from build123d import *

# Parameters (mm, degrees)
F0_W     = 205.775664
F0_H     = 100
F0_R     = 25
F1_DEPTH = 50
F2_W     = 20
F2_H     = 100
F3_DEPTH = 10
F5_DEPTH = 100.001
F6_R     = 7.5
F7_DEPTH = 25


with BuildPart() as f1:
    # F0 (on Top) → F1 (new body)
    with BuildSketch(Plane.XY):
        Rectangle(F0_W, F0_H)
        Circle(F0_R, mode=Mode.SUBTRACT)
    extrude(amount=F1_DEPTH)

    # F2 (on face) → F3 (cut)
    with BuildSketch(Plane(origin=(0, 0, 0), x_dir=(1, 0, 0), z_dir=(0, 0, -1))):
        with Locations((-67.887832, 0)):
            Rectangle(F2_W, F2_H)
        with BuildLine():
            Line((11, 50), (-11, 50))
            Line((-11, 50), (-11, 22.449944))
            ThreePointArc((-11, 22.449944), (0, 25), (11, 22.449944))
            Line((11, 22.449944), (11, 50))
        make_face()
        with BuildLine():
            Line((-11, -22.449944), (-11, -50))
            Line((-11, -50), (11, -50))
            Line((11, -50), (11, -22.449944))
            ThreePointArc((11, -22.449944), (0, -25), (-11, -22.449944))
        make_face()
    extrude(amount=-F3_DEPTH, mode=Mode.SUBTRACT)

    # F4 (on face) → F5 (cut, through all)
    with BuildSketch(Plane(origin=(0, 50, 0), x_dir=(-1, 0, 0), z_dir=(0, 1, 0))):
        Polygon((-62.5, 0), (-37.5, 0), (-31.726497, 10), (-68.273503, 10), align=None)
    extrude(amount=-F5_DEPTH, mode=Mode.SUBTRACT)

    # F6 (on face) → F7 (join)
    with BuildSketch(Plane.YZ.offset(102.887832)):
        with Locations((0, 25)):
            Circle(F6_R)
    extrude(amount=F7_DEPTH)


solid = f1.part
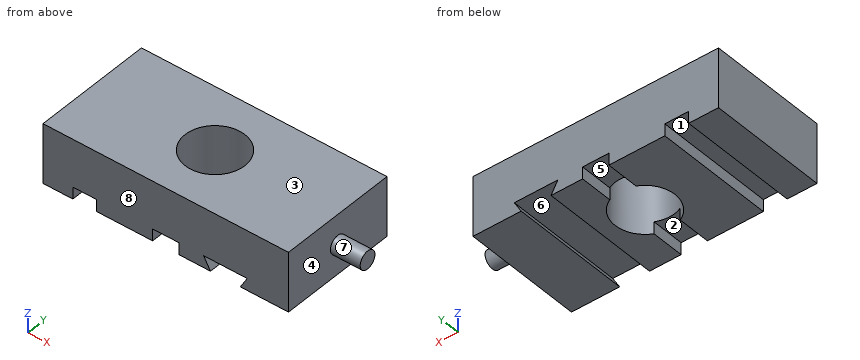
The listing builds one solid part. Answer for the finished solid, in the listing's coordinates (mm). Face numbers are marked on the shaded views. A direction names the side the tool comes from. Round coordinates to 2 decimals unless told otherwise and drop trailing zeros. Order: outer loops, then holes, each group sorted by start corner. A loop starts at its lowest first (then second) coordinate and runs counter-clockwise, first axis right, second up. Notation, with made-up numbers: (-14.75, 16.5) -> (0.25, 16.5) arc R12 cw to (0.25, 36.5) -> close; hole circle Ø1 at (86, 32.25). An arc over 180 degrees is marked (long way). Put each result on its own line as item: value.
Q1. Section D-D, the plane y = 42.5 is taken. Write down the section's boundary in (x, z).
Results list:
outline: (-102.89, 0) -> (-77.89, 0) -> (-77.89, 10) -> (-57.89, 10) -> (-57.89, 0) -> (-11, 0) -> (-11, 10) -> (11, 10) -> (11, 0) -> (37.5, 0) -> (31.73, 10) -> (68.27, 10) -> (62.5, 0) -> (102.89, 0) -> (102.89, 50) -> (-102.89, 50) -> close
Q2. Each of these flat-tipped pins is pushed along its axis until it touches: P1, Ø15, axis at y = 20.5, z = 17.5, coming from the +X side; P2, Ø1.5, axis at x = 40.5, y = -38, coming from the -Z side. Where does it stop, or does it pass through?
Results list:
P1: x = 102.89
P2: z = 10
Q3. Section A-A, the plane y = 0 is taken. Write down the section's boundary in (x, z).
Results list:
outline: (-102.89, 0) -> (-77.89, 0) -> (-77.89, 10) -> (-57.89, 10) -> (-57.89, 0) -> (-25, 0) -> (-25, 50) -> (-102.89, 50) -> close; (25, 0) -> (37.5, 0) -> (31.73, 10) -> (68.27, 10) -> (62.5, 0) -> (102.89, 0) -> (102.89, 17.5) -> (127.89, 17.5) -> (127.89, 32.5) -> (102.89, 32.5) -> (102.89, 50) -> (25, 50) -> close
Q4. Section B-B, the plane x = 0 is taken. Write down the section's boundary in (y, z), and give its area (3 significant figures).
Results list:
outline: (-50, 10) -> (-25, 10) -> (-25, 50) -> (-50, 50) -> close; (25, 10) -> (50, 10) -> (50, 50) -> (25, 50) -> close
area: 2,000 mm^2
Q5. Section C-C, the plane z = 25 is taken. Write down the section's boundary in (x, y).
Results list:
outline: (-102.89, -50) -> (102.89, -50) -> (102.89, -7.5) -> (127.89, -7.5) -> (127.89, 7.5) -> (102.89, 7.5) -> (102.89, 50) -> (-102.89, 50) -> close; hole circle Ø50 at (0, 0)
Q6. Which of the six approach directions +Z, -Z, +X, -X, +Y, -Y give full straight-line access (tool end or side, diameter ignored) to the marked faces 5, 6, 7 and 8?
Results list:
face 5: -Z, +Y, -Y
face 6: +Y, -Y
face 7: +X
face 8: +Z, -Z, +X, -X, -Y
Q7. Determine the mould class of the marked faces 1, 2, 3 and 4 for opening direction X: pulls with the +X half, pulls with the -X half, needs draft (parallel to the pull), parting line crosses it, or undercut.
Results list:
face 1: undercut
face 2: undercut
face 3: needs draft
face 4: pulls with the +X half
Q8. Consider line 1 along X through (y, z) = (0, 20.5); line 2 along X through (y, z) = (0, 17); line 3 along Y through (x, z) = (2.5, 47). Determine where each line is inside the solid, lowest interval first.
Results list:
line 1: -102.89 to -25, 25 to 127.89
line 2: -102.89 to -25, 25 to 102.89
line 3: -50 to -24.87, 24.87 to 50
